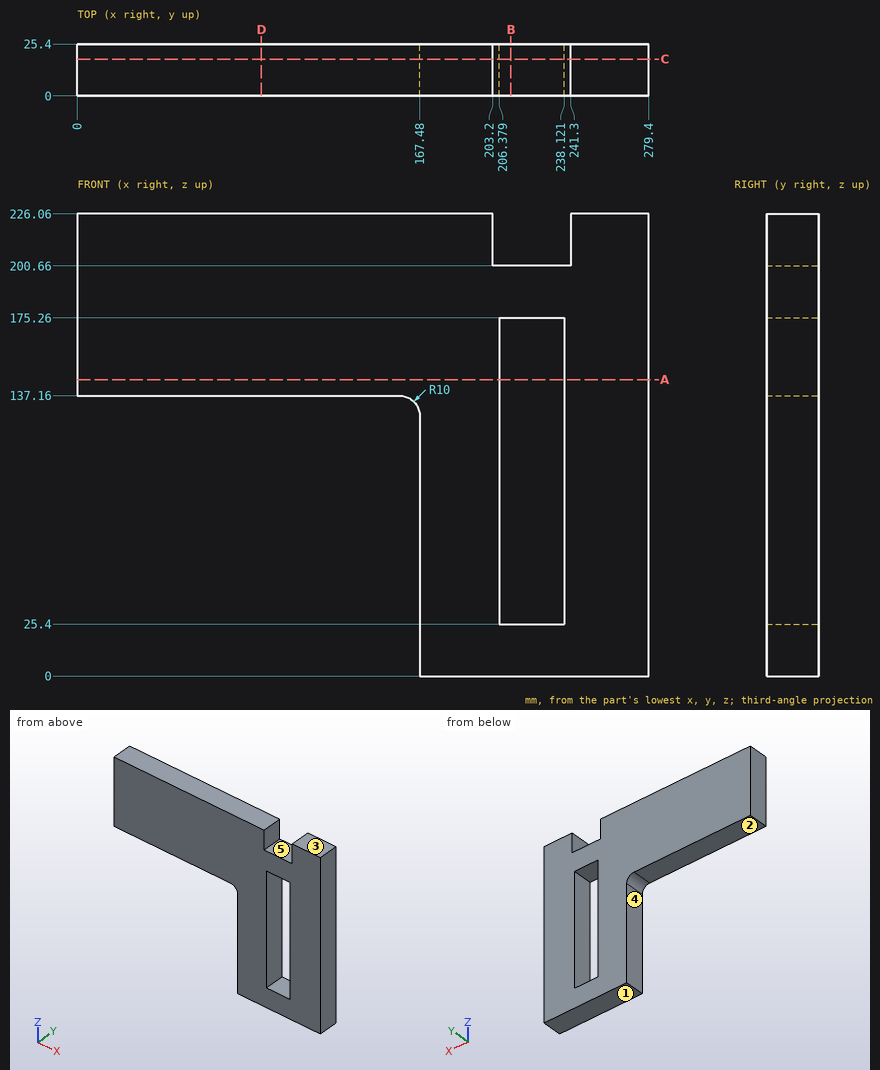
Answer from the drawing. Dimensions are ordinates in mm from the lowest x, y and z of the part. A direction names the side the tool comes from. Give positions to 0.01 mm unless a question says otherwise; leave off trailing zeros. Write each loop counter-clockwise with the first axis right and the second up, starting at its lowest first coordinate (ties: lowest second). Pieces come first, ordered by that corner, then holes. Notation, with made-up numbers: (-39, 6.25) -> (-15, 6.25) arc R20 cw to (-15, 14.25) -> close; hole circle Ø3 at (-25, 2). An arc over 180 degrees is marked (long way). Use a Markdown table: item, result.
(1) Section C-C, the plane y = 18 is taken. Determine the outline of the cut face in (x, z), then the cut area to 3 significant figures.
Return value:
| item | result |
|---|---|
| outline | (0, 137.16) -> (157.48, 137.16) arc R10 cw to (167.48, 127.16) -> (167.48, 0) -> (279.4, 0) -> (279.4, 226.06) -> (241.3, 226.06) -> (241.3, 200.66) -> (203.2, 200.66) -> (203.2, 226.06) -> (0, 226.06) -> close; hole (206.38, 25.4) -> (238.12, 25.4) -> (238.12, 175.26) -> (206.38, 175.26) -> close |
| area | 34,500 mm2 |
(2) Flat-ended cylindrical pins translate along their axes: P1, Ø12.5, axis at x = 218, y = 16, coming from the +Z side; P2, Ø10, axis at y = 21, z = 68.5, coming from the -X side; P3, Ø1.5, axis at x = 126.5, y = 13, coming from the -Z side. Find the tip coordinate at first contact, or state that the pin passes through.
Return value:
| item | result |
|---|---|
| P1 | z = 200.66 |
| P2 | x = 167.48 |
| P3 | z = 137.16 |
(3) For the marked faces 1 and 2, determine the directions among +Z, -Z, +X, -X, +Y, -Y from which every point of the face is accessible in a straight line to the end or side of a thin tool.
Return value:
| item | result |
|---|---|
| face 1 | -Z, +X, -X, +Y, -Y |
| face 2 | -Z, -X, +Y, -Y |
(4) Section B-B, the plane x = 212 is taken. Determine the outline of the cut face in (y, z).
Return value:
| item | result |
|---|---|
| outline | (0, 0) -> (25.4, 0) -> (25.4, 25.4) -> (0, 25.4) -> close; (0, 175.26) -> (25.4, 175.26) -> (25.4, 200.66) -> (0, 200.66) -> close |
(5) Section D-D, the plane x = 90 is taken. Determine the outline of the cut face in (y, z), then the cut area to 3 significant figures.
Return value:
| item | result |
|---|---|
| outline | (0, 137.16) -> (25.4, 137.16) -> (25.4, 226.06) -> (0, 226.06) -> close |
| area | 2,260 mm2 |
(6) Section A-A, the plane z = 145 is taken. Determine the outline of the cut face in (x, y), then the cut area to 3 significant figures.
Return value:
| item | result |
|---|---|
| outline | (0, 0) -> (206.38, 0) -> (206.38, 25.4) -> (0, 25.4) -> close; (238.12, 0) -> (279.4, 0) -> (279.4, 25.4) -> (238.12, 25.4) -> close |
| area | 6,290 mm2 |
(7) Determine the mould class of the marked faces 3, 4 and 5 for opening direction X: released by +X, released by -X, zero draft, split by the parting line, or undercut.
Return value:
| item | result |
|---|---|
| face 3 | zero draft |
| face 4 | released by -X |
| face 5 | undercut |
(8) Find the intervals of material crossed by probe 1 along X at (y, z) = (6, 170.5); probe 2 along X at (y, z) = (17.5, 51.5); probe 3 along Z at (x, y) = (219, 11.5), in increasing order. Write a range as from..to.
Return value:
| item | result |
|---|---|
| probe 1 | 0..206.38, 238.12..279.4 |
| probe 2 | 167.48..206.38, 238.12..279.4 |
| probe 3 | 0..25.4, 175.26..200.66 |
